Check sheet for the modelled part. Datum: model origin and axes. Units: mm. A direction names the side the tool comes from. Give positions to 0.01 mm unless a question says otherwise; leave off trailing zeros. Order: outer loops, then holes, each group sorted by start corner. A loop starts at its lowest first (then second) coordinate and runs counter-clockwise, first axis right, second up.
```python
from build123d import *

# Parameters (mm, degrees)
F0_R     = 9.525
F1_DEPTH = 25.4
F2_DEPTH = 25.4
F3_DEPTH = 12.0142


with BuildPart() as f1:
    # F0 (on Front) → F1 (new body)
    with BuildSketch(Plane.XZ):
        Circle(F0_R)
        Polygon((-4.7625, 0), (-4.7625, 4.7625), (0, 4.7625), (4.7625, 4.7625), (4.7625, 0), (4.7625, -4.7625), (0, -4.7625), (-4.7625, -4.7625), align=None, mode=Mode.SUBTRACT)
        with BuildLine():
            Line((4.7625, 4.7625), (0, 4.7625))
            ThreePointArc((0, 4.7625), (3.367596, 3.367596), (4.7625, 0))
            Line((4.7625, 0), (4.7625, 4.7625))
        make_face()
        with BuildLine():
            ThreePointArc((4.7625, 0), (3.367596, 3.367596), (0, 4.7625))
            ThreePointArc((0, 4.7625), (-3.367596, 3.367596), (-4.7625, 0))
            ThreePointArc((-4.7625, 0), (-3.367596, -3.367596), (0, -4.7625))
            ThreePointArc((0, -4.7625), (3.367596, -3.367596), (4.7625, 0))
        make_face()
        with BuildLine():
            ThreePointArc((0, -4.7625), (-3.367596, -3.367596), (-4.7625, 0))
            Line((-4.7625, 0), (-4.7625, -4.7625))
            Line((-4.7625, -4.7625), (0, -4.7625))
        make_face()
        with BuildLine():
            Line((4.7625, -4.7625), (4.7625, 0))
            ThreePointArc((4.7625, 0), (3.367596, -3.367596), (0, -4.7625))
            Line((0, -4.7625), (4.7625, -4.7625))
        make_face()
        with BuildLine():
            Line((0, 4.7625), (-4.7625, 4.7625))
            Line((-4.7625, 4.7625), (-4.7625, 0))
            ThreePointArc((-4.7625, 0), (-3.367596, 3.367596), (0, 4.7625))
        make_face()
    extrude(amount=F1_DEPTH)

    # F0 (on Front) → F2 (cut)
    with BuildSketch(Plane.XZ):
        with BuildLine():
            ThreePointArc((4.7625, 0), (3.367596, 3.367596), (0, 4.7625))
            ThreePointArc((0, 4.7625), (-3.367596, 3.367596), (-4.7625, 0))
            ThreePointArc((-4.7625, 0), (-3.367596, -3.367596), (0, -4.7625))
            ThreePointArc((0, -4.7625), (3.367596, -3.367596), (4.7625, 0))
        make_face()
    extrude(amount=F2_DEPTH, mode=Mode.SUBTRACT)

    # F0 (on Front) → F3 (cut)
    with BuildSketch(Plane.XZ):
        with BuildLine():
            ThreePointArc((0, -4.7625), (-3.367596, -3.367596), (-4.7625, 0))
            Line((-4.7625, 0), (-4.7625, -4.7625))
            Line((-4.7625, -4.7625), (0, -4.7625))
        make_face()
        with BuildLine():
            Line((4.7625, -4.7625), (4.7625, 0))
            ThreePointArc((4.7625, 0), (3.367596, -3.367596), (0, -4.7625))
            Line((0, -4.7625), (4.7625, -4.7625))
        make_face()
        with BuildLine():
            Line((0, 4.7625), (-4.7625, 4.7625))
            Line((-4.7625, 4.7625), (-4.7625, 0))
            ThreePointArc((-4.7625, 0), (-3.367596, 3.367596), (0, 4.7625))
        make_face()
        with BuildLine():
            Line((4.7625, 4.7625), (0, 4.7625))
            ThreePointArc((0, 4.7625), (3.367596, 3.367596), (4.7625, 0))
            Line((4.7625, 0), (4.7625, 4.7625))
        make_face()
    extrude(amount=F3_DEPTH, mode=Mode.SUBTRACT)


solid = f1.part
```
(1) Set-up check for faces 4 (the face through (-4.4, -25.4, 2.3)), 5 (the face through (0, -6, 4.762)): record each of +Z, -Z, +X, -X, +Y, -Y from which the full face is reachable in a straight line by a thin tool's end or side.
Response values:
face 4: +Z, -Z, +X, -X, -Y
face 5: +Y
(2) Cross-section at C-C on z = 1. Enter the section's corners in (x, y), then the cut area to 3 significant figures.
Response values:
outline: (-9.47, -25.4) - (-4.66, -25.4) - (-4.66, -12.01) - (-4.76, -12.01) - (-4.76, 0) - (-9.47, 0) - close; (4.66, -25.4) - (9.47, -25.4) - (9.47, 0) - (4.76, 0) - (4.76, -12.01) - (4.66, -12.01) - close
area: 242 mm2
(3) Cross-section at A-A on x = 0.75. Enter the section's corners in (y, z), then the cut area to 3 significant figures.
Response values:
outline: (-25.4, -9.5) - (0, -9.5) - (0, -4.76) - (-12.01, -4.76) - (-12.01, -4.7) - (-25.4, -4.7) - close; (-25.4, 4.7) - (-12.01, 4.7) - (-12.01, 4.76) - (0, 4.76) - (0, 9.5) - (-25.4, 9.5) - close
area: 242 mm2
(4) Release check for a two-part mould opening along Z. For faces 1 (the face through (0, 0, -6)), 2 (the face through (-7.559, -12.522, -5.796)), 3 (the face through (4, -12.014, -4)) record: released by +Z, released by -Z, zero draft, split by the parting line, or undercut.
Response values:
face 1: zero draft
face 2: split by the parting line
face 3: undercut
(5) Material ranges on L1, parallel to Z at x = 0.25, y = -2.75; L2, parallel to Z at x = 8.25, y = -24; L3, parallel to X at y = -1.5, z = 1.75, recorded low to high.
Response values:
L1: z = -9.52 to -4.76, 4.76 to 9.52
L2: z = -4.76 to 4.76
L3: x = -9.36 to -4.76, 4.76 to 9.36
(6) Gauge pin test, flat ends, axial feed: pin 1 Ø1 at (y, z) = (-19, -5) entering from +X (3 decimals); pin 2 Ø1 at (x, y) = (2.5, -21) entering from -Z; pin 3 Ø7.5 at (y, z) = (-5, -1.5) entering from -X (3 decimals); pin 4 Ø1 at (x, y) = (-4, -12.5) entering from -Z. Record the tip position at first contact, or that the pin passes through.
Response values:
pin 1: stops at x = 8.395
pin 2: stops at z = -9.31
pin 3: stops at x = -9.525
pin 4: stops at z = -8.86
